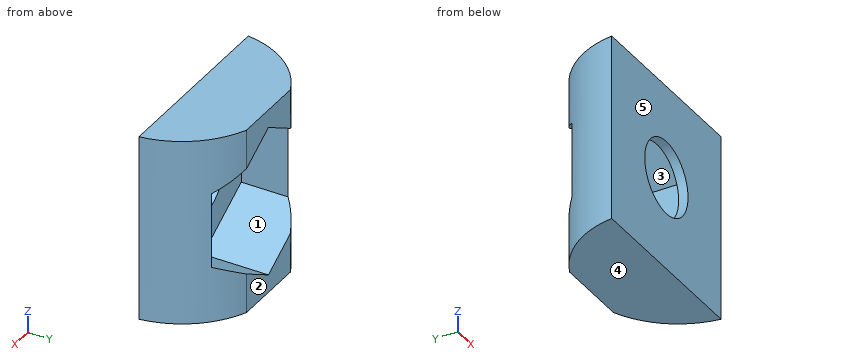
Autodesk Inventor part; units mm, degrees
ref_plane "YZ Plane" through (0, 0, 0) normal (1, 0, 0) x (0, 1, 0)
ref_plane "XZ Plane" through (0, 0, 0) normal (0, 1, 0) x (-1, 0, 0)
ref_plane "XY Plane" through (0, 0, 0) normal (0, 0, 1) x (1, 0, 0)
sketch "Sketch1" plane through (0, 0, 0) normal (0, 0, 1) x (1, 0, 0)
  line L0 (-5, 0) -> (5, 0)
  line L1 (0, 0) -> (0, 4) construction
  line L2 (-2, 4) -> (2, 4)
  arc A0 (-2, 4) -> (-5, 0) centre (-0.0359, -0.5981) ccw
  arc A1 (5, 0) -> (2, 4) centre (0.0359, -0.5981) ccw
  dimension "d0" = 10
  dimension "d1" = 4
  dimension "d2" = 4
  dimension "d3" = 5
  dimension "d4" = 5
extrude "Extrusion1" add sketch "Sketch1" along normal blind 10
sketch "Sketch2" plane through (-2, 4, 0) normal (0, 1, 0) x (1, 0, 0)
  circle A0 centre (2, -5) radius 1.975
  line L0 (4, 0) -> (0, 0)
  line L1 (0, 0) -> (0, -10)
  point P0 (2, 0)
  point P1 (2, 0)
  dimension "d7" = 3.95
  dimension "d8" = 5
  dimension "d9" = 2
extrude "Extrusion2" cut sketch "Sketch2" against normal blind 10
sketch "Sketch3" plane through (-2, 4, 0) normal (0, 1, 0) x (1, 0, 0)
  point P0 (2, 0)
sketch "Sketch5" plane through (-2, 4, 0) normal (0, 1, 0) x (1, 0, 0)
  circle A0 centre (2, -5) radius 1.975
  line L0 (2, -0.9585) -> (5.5, -2.9793)
  line L1 (5.5, -2.9793) -> (5.5, -7.0207)
  line L2 (5.5, -7.0207) -> (2, -9.0415)
  line L3 (2, -9.0415) -> (-1.5, -7.0207)
  line L4 (-1.5, -7.0207) -> (-1.5, -2.9793)
  line L5 (-1.5, -2.9793) -> (2, -0.9585)
  point P0 (2, 0)
  point P1 (5.5, -5)
  dimension "d15" = 3.5
extrude "Extrusion4" cut sketch "Sketch5" against normal blind 3.5
properties part number "RailNut"
The listing builds one solid part. Answer for the finished solid, in the listing's coordinates (mm). Face numbers are marked on the shaded views. A direction names the side the tool comes from. Coordinates: 2 decimals unless noted, no trailing zeros. Write each loop counter-clockwise with the first axis right and the second up, starting at its lowest first coordinate (ties: lowest second). Pieces come first, ordered by that corner, then holes. Notation, with made-up numbers: (64.5, 57.5) - (123.5, 57.5) arc R23 cw to (123.5, 73.5) - close; hole circle Ø8 at (6.25, -2). An arc over 180 degrees is marked (long way). Return JSON: item names as keys, results as strings.
1. The part is cut by section B-B on y = 3.55. Determine the outline of the cut face in (x, z), then the cut area to 3 significant figures.
Final values:
{"outline": "(-2.83, 0) - (2.83, 0) - (2.83, 2.59) - (0, 0.96) - (-2.83, 2.59) - close; (-2.83, 7.41) - (0, 9.04) - (2.83, 7.41) - (2.83, 10) - (-2.83, 10) - close", "area": "20.1 mm^2"}
2. Which of the six approach directions +Z, -Z, +X, -X, +Y, -Y give full straight-line access (tool end or side, diameter ignored) to the marked faces 1 and 2?
Final values:
{"face 1": "+Y", "face 2": "+Z, -Z, +X, -X, +Y"}
3. The part is cut by section C-C on x = 1. Determine the outline of the cut face in (y, z), then the cut area to 3 significant figures.
Final values:
{"outline": "(0, 0) - (4, 0) - (4, 1.54) - (0.5, 1.54) - (0.5, 3.3) - (0, 3.3) - close; (0, 6.7) - (0.5, 6.7) - (0.5, 8.46) - (4, 8.46) - (4, 10) - (0, 10) - close", "area": "14.0 mm^2"}
4. The part is cut by section A-A on z = 5. Determine the outline of the cut face in (x, y) (3 decimals), then the cut area to 3 significant figures.
Final values:
{"outline": "(-5, 0) - (-1.975, 0) - (-1.975, 0.5) - (-3.5, 0.5) - (-3.5, 3.007) arc R5 ccw to start; (1.975, 0) - (5, 0) arc R5 ccw to (3.5, 3.007) - (3.5, 0.5) - (1.975, 0.5) - close", "area": "7.35 mm^2"}
5. For a pull along Z with two mould halves and no side action, classify the marked faces 3, 4 and 5 as +Z half, -Z half, draft (parallel to the pull), parting line (faces both ways), or undercut.
Final values:
{"face 3": "undercut", "face 4": "-Z half", "face 5": "draft"}
6. Consider line 1 along Z through (x, y) = (0, 0.3) (3 decimals); line 2 along Y through (x, z) = (2.5, 2.5); line 3 along Z through (x, y) = (0.25, 3.3). Determine where each line is inside the solid, lowest interval first.
Final values:
{"line 1": "0 to 3.025, 6.975 to 10", "line 2": "0 to 0.5", "line 3": "0 to 1.1, 8.9 to 10"}
7. The part is cut by section D-D on x = -2.25. Determine the outline of the cut face in (y, z), then the cut area to 3 significant figures.
Final values:
{"outline": "(0, 0) - (3.88, 0) - (3.88, 2.26) - (0.5, 2.26) - (0.5, 7.74) - (3.88, 7.74) - (3.88, 10) - (0, 10) - close", "area": "20.3 mm^2"}
8. Each of these flat-tipped pins is pushed along its axis until it touches: pin 1 Ø2 at (y, z) = (1, 4) entering from -X; pin 2 Ø2 at (y, z) = (2, 5.5) entering from +X; pin 3 Ø2.5 at (x, z) = (0, 5) entering from -Y; pin 4 Ø3.5 at (x, z) = (1, 4.5) entering from +Y. Where does it stop, or does it pass through?
Final values:
{"pin 1": "x = -5", "pin 2": "x = 4.77", "pin 3": "through", "pin 4": "y = 0.5"}
